Verification items for this drawing (mm, ordinates from the low corner). Round coordinates to 2 decimals unless told otherwise and drop trailing zeros. Write each loop counter-clockwise with the first axis right and the second up, starting at its lowest first coordinate (ties: lowest second). Pieces come first, ordered by that corner, then holes. Notation, with made-up numbers: (83.25, 44.5) -> (122.25, 44.5) arc R19 ccw to (122.25, 81.5) -> close; hole circle Ø4 at (41, 78.25). An arc over 180 degrees is marked (long way). One line per question, with ' | ' between items.
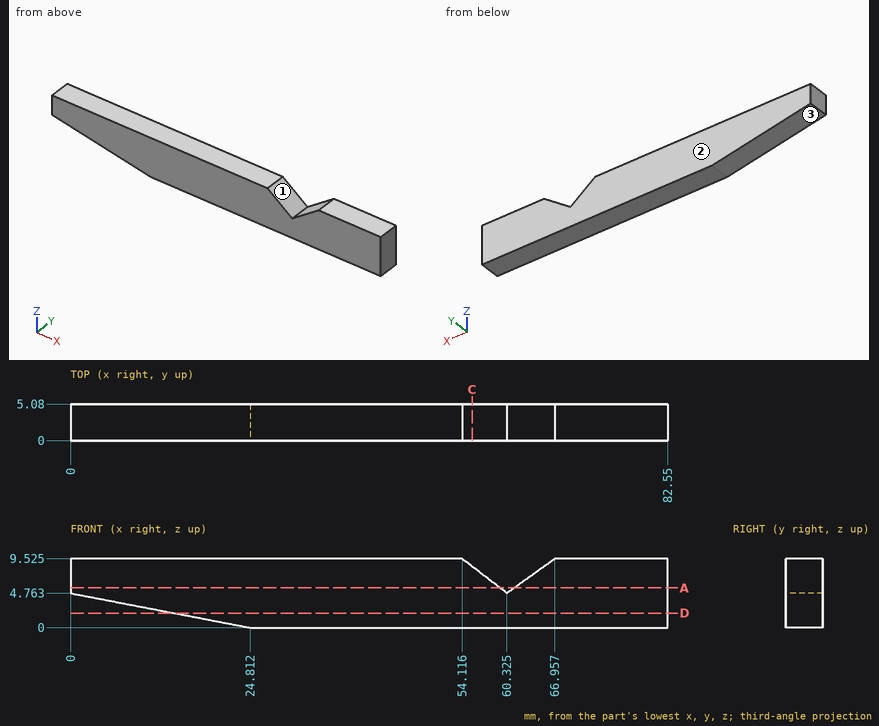
(1) Draft check along X on the marked faces 1, 2 and 3. Enter one of: +X half, -X half, draft (parallel to the pull), parting line (faces both ways), or undercut.
Resolved:
face 1: undercut | face 2: draft | face 3: -X half
(2) Sectioned sample at C-C on x = 55.5. Record the cut outline in (y, z), then the cut area to 3 significant figures.
Resolved:
outline: (0, 0) -> (5.08, 0) -> (5.08, 8.46) -> (0, 8.46) -> close | area: 43.0 mm2
(3) Sectioned sample at A-A on z = 5.5. Record the cut outline in (x, y).
Resolved:
outline: (0, 0) -> (59.36, 0) -> (59.36, 5.08) -> (0, 5.08) -> close; (61.35, 0) -> (82.55, 0) -> (82.55, 5.08) -> (61.35, 5.08) -> close
(4) Go/stop test with a flat-tipped pin: pin 1 (3 mm diameter, centred on x = 67, y = 1.5, fed in from -Z). Record where the tip stops, or that it passes through.
Resolved:
pin 1: stops at z = 0
(5) Sectioned sample at D-D on z = 2. Record the cut outline in (x, y).
Resolved:
outline: (14.39, 0) -> (82.55, 0) -> (82.55, 5.08) -> (14.39, 5.08) -> close
(6) Material ranges on line 1 (Z direction, x = 62, y = 2.5) (1 decimal); line 2 (Z direction, x = 59.5, y = 0.5) (1 decimal), recorded low to high.
Resolved:
line 1: z = 0 to 6 | line 2: z = 0 to 5.4
